Part model, mm, in its own coordinate system. A direction names the side the tool comes from. Round coordinates to 2 decimals unless told otherwise and drop trailing zeros. Loops run counter-clockwise (first coordinate to the right, second up) from the corner with the lowest first, then second, coordinate; pieces in that order, holes last. Notation, with made-up numbers: (80.5, 68) -> (112.5, 68) arc R23 cw to (112.5, 76) -> close; hole circle Ø5 at (-15.75, -23). An arc over 180 degrees is marked (long way). Use a Markdown table: item, result. Add a question column.
Item 1: Probe line 1 (X direction, y = 23.5, z = 0); line 2 (X direction, y = 7, z = -18); line 3 (X direction, y = 15, z = -9.5). List the from-to ranges inside material, lowest first. Write a range as [from, to].
Item 2: Cut at A-A, the plane x = 0. List the corners of the cut face in (y, z).
Item 3: Cut at C-C, the plane y = 25. State how many separate pieces and enclosed holes the cut face has, plus the area to 3 significant figures.
Item 4: Two-plate mould, pull along Y, no slides. Class faces 5 (the face through (21.3, 39.37, -14.3)), 6 (the face through (-39, 16, -12.7)), 7 (the face through (44, 5.588, -16)): pulls with the +Y half, pulls with the -Y half, needs draft (parallel to the pull), parting line crosses it, or undercut.
Item 5: Flat gauge pins, fed straight in: pin 1 (12 mm diameter, centred on x = -37.5, y = 20, fed in from +Z); pin 2 (3 mm diameter, centred on x = 51.5, y = 12, fed in from -Z); pin 3 (2 mm diameter, centred on x = 34, z = 18.5, fed in from +Y). Where does each tip first touch, or does it go through?
Item 6: Which spindle directions (+Z, -Z, +X, -X, +Y, -Y) get a long thin tool onto all of the face, cutting with end or side? Do faces 1 (the face through (47, 20, 19.05)), 2 (the face through (41.771, 17, -16)), 3 (the face through (46, 20, -19.05)), 4 (the face through (-46.99, 16, 11)). Say none if no direction does.
Item 7: Cut at D-D, the plane z = 39.5. List the corners of the cut face in (x, y), plus the area to 3 significant figures.
```python
from build123d import *

# Parameters (mm, degrees)
SKETCH1_R           = 44.069
BOSS_EXTRUDE1_DEPTH = 40.64
SKETCH2_R           = 44.069
SKETCH2_R_2         = 41.402
BOSS_EXTRUDE2_DEPTH = 1.2954
BOSS_EXTRUDE3_DEPTH = 38.1
CUT_EXTRUDE1_DEPTH  = 31.75
SKETCH5_W           = 3.81
SKETCH5_H           = 22.86
CUT_EXTRUDE2_DEPTH  = 93.670068167
FILLET1_R           = 2.54
SKETCH7_R           = 25.4
CUT_EXTRUDE3_DEPTH  = 27.94
SKETCH8_R           = 11.43
CUT_EXTRUDE4_DEPTH  = 81.906181129
SKETCH9_R           = 31.75
CUT_EXTRUDE5_DEPTH  = 1.27


with BuildPart() as part:
    # Sketch1 → Boss-Extrude1 (new body)
    with BuildSketch(Plane(origin=(0, 0, 0), x_dir=(1, 0, 0), z_dir=(0, 1, 0))):
        with Locations(Location((0, 0, 0), (0, 0, 270))):
            Circle(SKETCH1_R)
    extrude(amount=BOSS_EXTRUDE1_DEPTH)

    # Sketch2 → Boss-Extrude2 (add)
    with BuildSketch(Plane(origin=(0, 40.64, 0), x_dir=(1, 0, 0), z_dir=(0, 1, 0))):
        with Locations(Location((0, 0, 0), (0, 0, 270))):
            Circle(SKETCH2_R)
        with Locations(Location((0, 0, 0), (0, 0, 270))):
            Circle(SKETCH2_R_2, mode=Mode.SUBTRACT)
    extrude(amount=BOSS_EXTRUDE2_DEPTH)

    # Sketch3 → Boss-Extrude3 (add)
    with BuildSketch(Plane(origin=(0, 0, 0), x_dir=(1, 0, 0), z_dir=(0, 1, 0))):
        with BuildLine():
            ThreePointArc((39.738825612, -19.05), (44.069, 0), (39.738825612, 19.05))
            Line((39.738825612, 19.05), (53.34, 19.05))
            Line((53.34, 19.05), (53.34, -19.05))
            Line((53.34, -19.05), (39.738825612, -19.05))
        make_face()
        with BuildLine():
            ThreePointArc((-39.738825612, 19.05), (-44.069, 0), (-39.738825612, -19.05))
            Line((-39.738825612, -19.05), (-53.34, -19.05))
            Line((-53.34, -19.05), (-53.34, 19.05))
            Line((-53.34, 19.05), (-39.738825612, 19.05))
        make_face()
    extrude(amount=BOSS_EXTRUDE3_DEPTH)

    # Sketch4 → Cut-Extrude1 (cut)
    with BuildSketch(Plane(origin=(0, 0, 0), x_dir=(1, 0, 0), z_dir=(0, 1, 0))):
        Polygon((-53.34, -8.89), (-53.34, 8.89), (-46.99, 8.89), (-46.99, 12.7), (-31.75, 12.7), (-31.75, -12.7), (-46.99, -12.7), (-46.99, -8.89), align=None)
        Polygon((46.99, -12.7), (46.99, -8.89), (53.34, -8.89), (53.34, 8.89), (46.99, 8.89), (46.99, 12.7), (31.75, 12.7), (31.75, -12.7), align=None)
    extrude(amount=CUT_EXTRUDE1_DEPTH, mode=Mode.SUBTRACT)

    # Sketch5 → Cut-Extrude2 (cut, through all)
    with BuildSketch(Plane(origin=(0, 0, -19.05), x_dir=(-1, 0, 0), z_dir=(0, 0, -1))):
        with Locations((43.675825612, 17.018)):
            Rectangle(SKETCH5_W, SKETCH5_H)
        with Locations((-43.675825612, 17.018)):
            Rectangle(SKETCH5_W, SKETCH5_H)
    extrude(amount=-CUT_EXTRUDE2_DEPTH, mode=Mode.SUBTRACT)

    # Fillet1
    fillet1_edges = [part.edges().sort_by_distance(p)[0] for p in [
        (44.069, 38.1, 0),
        (-44.069, 38.1, 0),
    ]]
    fillet(fillet1_edges, radius=FILLET1_R)

    # Sketch7 → Cut-Extrude3 (cut)
    with BuildSketch(Plane(origin=(0, 40.64, 0), x_dir=(1, 0, 0), z_dir=(0, 1, 0))):
        with Locations(Location((0, 0, 0), (0, 0, 270))):
            Circle(SKETCH7_R)
    extrude(amount=-CUT_EXTRUDE3_DEPTH, mode=Mode.SUBTRACT)

    # Sketch8 → Cut-Extrude4 (cut, through all)
    with BuildSketch(Plane.XZ):
        with Locations(Location((0, 0, 0), (0, 0, 270))):
            Circle(SKETCH8_R)
    extrude(amount=-CUT_EXTRUDE4_DEPTH, mode=Mode.SUBTRACT)

    # Sketch9 → Cut-Extrude5 (cut)
    with BuildSketch(Plane(origin=(0, 40.64, 0), x_dir=(1, 0, 0), z_dir=(0, 1, 0))):
        with Locations(Location((0, 0, 0), (0, 0, 270))):
            Circle(SKETCH9_R)
    extrude(amount=-CUT_EXTRUDE5_DEPTH, mode=Mode.SUBTRACT)


solid = part.part
```
A:
| question | item | result |
|---|---|---|
| 1 | line 1 | x = [-31.75, -25.4], [25.4, 31.75] |
| 1 | line 2 | x = [-53.34, -45.58], [-41.77, 41.77], [45.58, 53.34] |
| 1 | line 3 | x = [-53.34, -46.99], [-31.75, -23.56], [23.56, 31.75], [46.99, 53.34] |
| 2 | outline | (0, -44.07) -> (41.94, -44.07) -> (41.94, -41.4) -> (40.64, -41.4) -> (40.64, -31.75) -> (39.37, -31.75) -> (39.37, -25.4) -> (12.7, -25.4) -> (12.7, -11.43) -> (0, -11.43) -> close; (0, 11.43) -> (12.7, 11.43) -> (12.7, 25.4) -> (39.37, 25.4) -> (39.37, 31.75) -> (40.64, 31.75) -> (40.64, 41.4) -> (41.94, 41.4) -> (41.94, 44.07) -> (0, 44.07) -> close |
| 3 | separate pieces | 5 |
| 3 | enclosed holes | 1 |
| 3 | area | 3,790 mm^2 |
| 4 | face 5 | pulls with the +Y half |
| 4 | face 6 | needs draft |
| 4 | face 7 | undercut |
| 5 | pin 1 | stops at z = 30.82 |
| 5 | pin 2 | stops at z = -19.05 |
| 5 | pin 3 | stops at y = 40.64 |
| 6 | face 1 | +Z, +X, +Y, -Y |
| 6 | face 2 | +Z, -Z |
| 6 | face 3 | -Z, +X, +Y, -Y |
| 6 | face 4 | -Y |
| 7 | outline | (-19.54, 0) -> (19.54, 0) -> (19.54, 41.94) -> (12.4, 41.94) -> (12.4, 40.64) -> (-12.4, 40.64) -> (-12.4, 41.94) -> (-19.54, 41.94) -> close |
| 7 | area | 1,610 mm^2 |
